Drawing for the job (mm, zero at the part's lowest x, y, z). Give positions to 0.01 mm unless a question says otherwise; leave off trailing zeros. Order: outer loops, then holes, each group sorted by start corner. A loop starts at its lowest first (then second) coordinate and runs counter-clockwise, first axis right, second up. Notation, with made-up numbers: M 78.25,6 L 110.25,6 A20 cw 110.25,14 Z; hole C 52.25,-31 d7. An arc over 180 degrees is marked long. One line per item, written item: value.
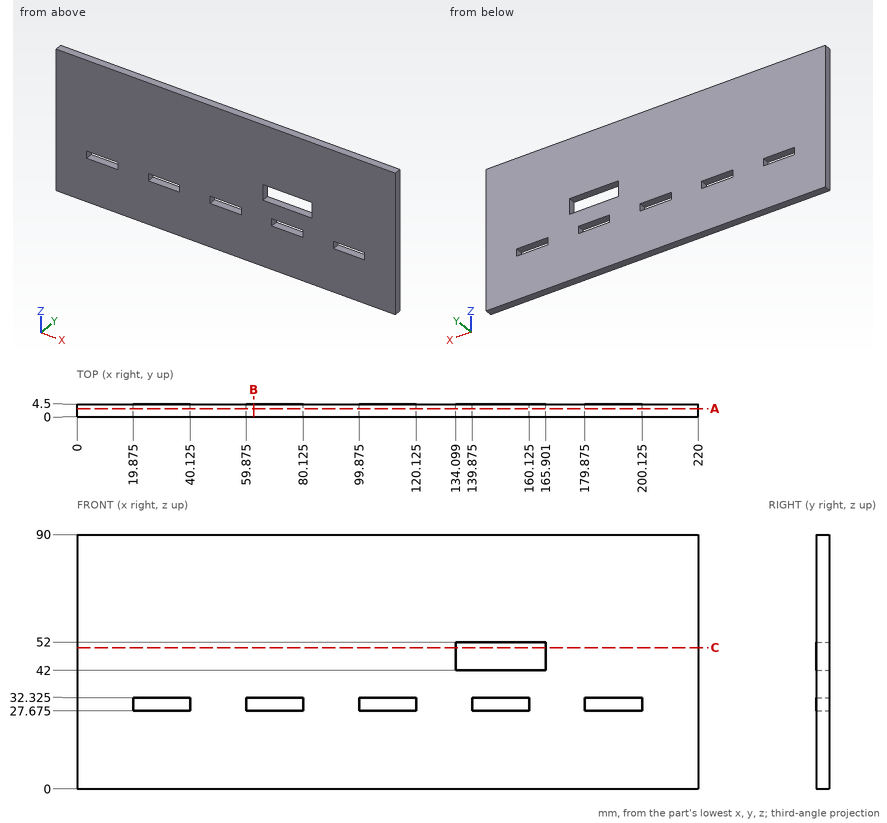
1) Saw through at A-A, the plane y = 2.85. Write the cut outline in (x, z) (1 decimal).
Check values:
outline: M 0,0 L 220,0 L 220,90 L 0,90 Z; hole M 19.9,27.7 L 40.1,27.7 L 40.1,32.3 L 19.9,32.3 Z; hole M 59.9,27.7 L 80.1,27.7 L 80.1,32.3 L 59.9,32.3 Z; hole M 99.9,27.7 L 120.1,27.7 L 120.1,32.3 L 99.9,32.3 Z; hole M 134.1,42 L 165.9,42 L 165.9,52 L 134.1,52 Z; hole M 139.9,27.7 L 160.1,27.7 L 160.1,32.3 L 139.9,32.3 Z; hole M 179.9,27.7 L 200.1,27.7 L 200.1,32.3 L 179.9,32.3 Z
2) Saw through at C-C, the plane z = 50. Write the cut outline in (x, y), then the cut area to 3 significant figures.
Check values:
outline: M 0,0 L 134.1,0 L 134.1,4.5 L 0,4.5 Z; M 165.9,0 L 220,0 L 220,4.5 L 165.9,4.5 Z
area: 847 mm^2
3) Saw through at B-B, the plane x = 62.5. Write the cut outline in (y, z) (1 decimal), then the cut area to 3 significant figures.
Check values:
outline: M 0,0 L 4.5,0 L 4.5,27.7 L 0,27.7 Z; M 0,32.3 L 4.5,32.3 L 4.5,90 L 0,90 Z
area: 384 mm^2
4) Drill centre lines: probe 1 along Z at (x, y) = (71.5, 0.95) (1 decimal); probe 2 along X at (y, z) = (1.7, 29.5) (1 decimal); probe 3 along X at (y, z) = (2.8, 45.5). Where is each one in solid material? Low to high. Write a range as from..to.
Check values:
probe 1: 0..27.7, 32.3..90
probe 2: 0..19.9, 40.1..59.9, 80.1..99.9, 120.1..139.9, 160.1..179.9, 200.1..220
probe 3: 0..134.1, 165.9..220
